Geometry check sheet. Reference: the model listing, model coordinates, mm. Face numbers are marked on the shaded views. A direction names the side the tool comes from. Give positions to 0.01 mm unless a question says otherwise; leave off trailing zeros. Order: outer loops, then holes, each group sorted by start corner. A loop starts at its lowest first (then second) coordinate and runs counter-clockwise, first axis right, second up. Notation, with made-up numbers: M -14.5,-11.5 L -8.5,-11.5 A12 ccw -8.5,4.5 Z; hole C 51,21 d6. An arc over 180 degrees is marked long. Answer as a JSON object with one key per item and string values. Group by question number.
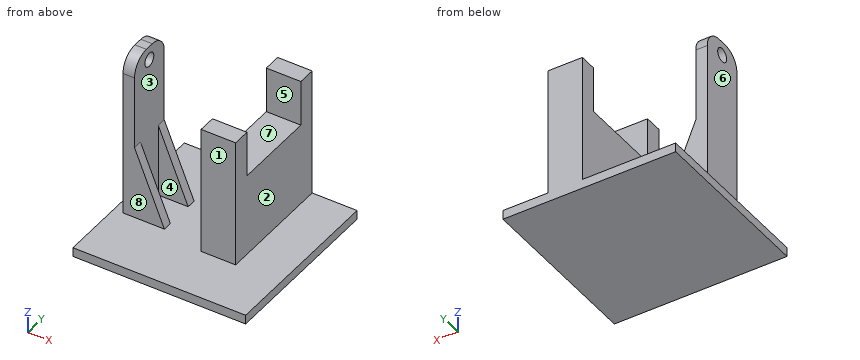
from build123d import *

# Parameters (mm, degrees)
F0_W      = 47.625
F0_H      = 47.625
F1_DEPTH  = 2.54
F3_W      = 9.525
F3_H      = 32.7025
F4_DEPTH  = 22.86
F5_W      = 9.525
F5_H      = 4.826
F6_DEPTH  = 12.7
F7_W      = 3.175
F7_H      = 12.7
F8_DEPTH  = 45.72
F9_R      = 1.905
F10_DEPTH = 25.4
F11_R     = 5.08
F13_DEPTH = 2.54


# Not quite as in the source:
# - a pattern or mirror of a feature is missing from the dataset's text; its kind, count and spacing are read off the source's solid


with BuildPart() as f1:
    # F0 (on Top) → F1 (new body)
    with BuildSketch(Plane.XY):
        Rectangle(F0_W, F0_H)
    extrude(amount=F1_DEPTH)

    # F3 (on face) → F4 (join)
    with BuildSketch(Plane.XY.offset(2.54)):
        with Locations((6.6675, 7.46125)):
            Rectangle(F3_W, F3_H)
    extrude(amount=F4_DEPTH)

    # F5 (on face) → F6 (join)
    with BuildSketch(Plane.XY.offset(25.4)):
        with Locations((6.6675, -6.477)):
            Rectangle(F5_W, F5_H)
        with Locations((6.6675, 21.3995)):
            Rectangle(F5_W, F5_H)
    extrude(amount=F6_DEPTH)

    # F7 (on face) → F8 (join)
    with BuildSketch(Plane.XY.offset(2.54)):
        with Locations((-19.685, 0)):
            Rectangle(F7_W, F7_H)
    extrude(amount=F8_DEPTH)

    # F9 (on face) → F10 (cut)
    with BuildSketch(Plane.YZ.offset(-18.0975)):
        with Locations((0, 44.45)):
            Circle(F9_R)
    extrude(amount=-F10_DEPTH, mode=Mode.SUBTRACT)

    # F11
    f11_edges = [f1.edges().sort_by_distance(p)[0] for p in [
        (-19.685, 6.35, 48.26),
        (-19.685, -6.35, 48.26),
    ]]
    fillet(f11_edges, radius=F11_R)

    # F12 (on face) → F13 (join)
    with BuildSketch(Plane(origin=(0, 6.35, 0), x_dir=(-1, 0, 0), z_dir=(0, 1, 0))):
        Polygon((18.0975, 2.54), (18.0975, 22.86), (9.8562051214, 2.54), align=None)
    f13 = extrude(amount=-F13_DEPTH)

    # F13_copies: F13 across plane
    add(f13.mirror(Plane(origin=(0, 0, 0), x_dir=(0, 0, -1), z_dir=(0, -1, 0))))


solid = f1.part
1. Cross-section at D-D (y = 8). Record the cut outline in (x, z) (1 decimal), and give its area (3 significant figures).
2. Depth check by flat-ended pin: pin 1 (4 mm diameter, centred on x = -12.5, z = 14.5, fed in from +Y); pin 2 (4 mm diameter, centred on x = -14.5, y = -2, fed in from -Z); pin 3 (5.5 mm diameter, centred on x = -14.5, z = 15, fed in from -Y); pin 4 (10.5 mm diameter, centred on x = 6, z = 33.5, fed in from -Y). Enter the tip coordinate at first touch or a pass-through.
3. Cross-section at A-A (z = 27). State how many separate pieces and enclosed holes the cut face has, and give its area (3 significant figures).
4. Access from +Z, -Z, +X, -X, +Y, -Y to the whole of each face (thin tool, end or side, straight path). Record for the marked faces 4, 5, 6, 7 and 8.
5. Thickness scan on line 1 along X through (y, z) = (-1, 7) (1 decimal); line 2 along Z through (x, y) = (-19.4, 0) (3 decimals); line 3 along X through (y, z) = (3, 42.5). Record the ranges inside material, lowest first. Write a range as [from, to].
6. Cross-section at B-B (y = 0). Record the cut outline in (x, z) (1 decimal).
7. Release check for a two-part mould opening along X. For the marked faces 1, 2 and 3 record: released by +X, released by -X, zero draft, split by the parting line, or undercut.
Report:
{
 "1": {"outline": "M -23.8,0 L 23.8,0 L 23.8,2.5 L 11.4,2.5 L 11.4,25.4 L 1.9,25.4 L 1.9,2.5 L -23.8,2.5 Z", "area": "339 mm2"},
 "2": {"pin 1": "passes through", "pin 2": "stops at z = 0", "pin 3": "stops at y = -6.35", "pin 4": "stops at y = -8.89"},
 "3": {"separate pieces": "3", "enclosed holes": "0", "area": "132 mm2"},
 "4": {"face 4": "+Z", "face 5": "+Z, +X, -X", "face 6": "+Z, -X, +Y, -Y", "face 7": "+Z, +X", "face 8": "+Z, -X, -Y"},
 "5": {"line 1": "x = [-21.3, -18.1], [1.9, 11.4]", "line 2": "z = [0, 42.545], [46.355, 48.26]", "line 3": "x = [-21.27, -18.1]"},
 "6": {"outline": "M -23.8,0 L 23.8,0 L 23.8,2.5 L 11.4,2.5 L 11.4,25.4 L 1.9,25.4 L 1.9,2.5 L -18.1,2.5 L -18.1,42.5 L -21.3,42.5 L -21.3,2.5 L -23.8,2.5 Z; M -21.3,46.4 L -18.1,46.4 L -18.1,48.3 L -21.3,48.3 Z"},
 "7": {"face 1": "zero draft", "face 2": "released by +X", "face 3": "undercut"}
}
